from build123d import *
from OCP.BRepAlgoAPI import BRepAlgoAPI_Cut
from OCP.TopTools import TopTools_ListOfShape
from build123d.topology import SkipClean

# Parameters (mm, degrees)
BOSS_EXTRUDE1_DEPTH = 7.5
CUT_EXTRUDE1_DEPTH  = 3.2
CUT_EXTRUDE4_REACH  = 70.655
SKETCH5_W           = 3
SKETCH5_H           = 17
CUT_EXTRUDE5_REACH  = 70.655
SKETCH8_W           = 12
SKETCH8_H           = 37
CUT_EXTRUDE6_DEPTH  = 3.2
SKETCH10_W          = 10
SKETCH10_H          = 7.5
BOSS_EXTRUDE2_DEPTH = 27.486353186
SKETCH11_W          = 3
SKETCH11_H          = 7.5
CUT_EXTRUDE7_DEPTH  = 3.5
SKETCH12_W          = 2
SKETCH12_H          = 7.5
CUT_EXTRUDE8_DEPTH  = 4
SKETCH13_W          = 2
SKETCH13_H          = 7.5
CUT_EXTRUDE9_DEPTH  = 4
SKETCH14_W          = 7.5
SKETCH14_H          = 9.5
CUT_EXTRUDE10_DEPTH = 6
SKETCH15_W          = 1.5
SKETCH15_H          = 21
SKETCH15_H_2        = 1
CUT_EXTRUDE11_DEPTH = 1.5
SKETCH16_W          = 1.5
SKETCH16_H          = 7.5
CUT_EXTRUDE12_DEPTH = 35.486360958
CUT_EXTRUDE13_DEPTH = 6
SKETCH19_W          = 17.5
SKETCH19_H          = 32
BOSS_EXTRUDE3_DEPTH = 7.5
CUT_EXTRUDE14_DEPTH = 6
SKETCH20_W          = 18
SKETCH20_H          = 6
CUT_EXTRUDE15_DEPTH = 6
SKETCH21_W          = 20
SKETCH21_H          = 33
CUT_EXTRUDE16_DEPTH = 11
CUT_EXTRUDE17_DEPTH = 5
CUT_EXTRUDE18_DEPTH = 10
SKETCH23_W          = 50
SKETCH23_H          = 4
BOSS_EXTRUDE4_DEPTH = 15
SKETCH25_R          = 3.5
CUT_EXTRUDE19_DEPTH = 10


with BuildPart() as part:
    # Sketch1 → Boss-Extrude1 (new body)
    with BuildSketch(Plane.XY):
        with BuildLine():
            Line((-33, -47.5), (49, -47.5))
            Line((49, -47.5), (49, -29.5))
            Line((49, -29.5), (31.5, -29.5))
            Line((31.5, -29.5), (31.5, 2.5))
            Line((31.5, 2.5), (49, 2.5))
            Line((49, 2.5), (49, 47.5))
            Line((49, 47.5), (30, 47.5))
            Line((30, 47.5), (30, 30.5))
            Line((30, 30.5), (27, 30.5))
            Line((27, 30.5), (27, 47.5))
            Line((27, 47.5), (-49, 47.5))
            Line((-49, 47.5), (-49, -31.5))
            ThreePointArc((-49, -31.5), (-44.313708499, -42.813708499), (-33, -47.5))
        make_face()
    extrude(amount=BOSS_EXTRUDE1_DEPTH)

    # Sketch2 → Cut-Extrude1 (cut)
    with BuildSketch(Plane.XY.offset(7.5)):
        Polygon((30, 40), (31, 40), (31, 32.5), (36, 32.5), (36, 28.5), (38, 28.5), (38, 32.5), (48, 32.5), (48, 46.5), (38, 46.5), (38, 47.5), (36, 47.5), (36, 46.5), (31, 46.5), (31, 45), (30, 45), align=None)
        Polygon((-16, 40), (-15, 40), (-15, 32.5), (-10, 32.5), (-10, 28.5), (-8, 28.5), (-8, 32.5), (2, 32.5), (2, 46.5), (-8, 46.5), (-8, 47.5), (-10, 47.5), (-10, 46.5), (-15, 46.5), (-15, 45), (-16, 45), align=None)
        Polygon((7, 40), (8, 40), (8, 32.5), (13, 32.5), (13, 28.5), (15, 28.5), (15, 32.5), (25, 32.5), (25, 46.5), (15, 46.5), (15, 47.5), (13, 47.5), (13, 46.5), (8, 46.5), (8, 45), (7, 45), align=None)
    extrude(amount=-CUT_EXTRUDE1_DEPTH, mode=Mode.SUBTRACT)

    # Sketch5 → Cut-Extrude4 (cut, up to next)
    with BuildSketch(Plane.XY.offset(7.5), mode=Mode.PRIVATE) as cut_extrude4_sk1:
        with Locations((5.5, 39)):
            Rectangle(SKETCH5_W, SKETCH5_H)
    cut_extrude4_tool1 = extrude(cut_extrude4_sk1.sketch, amount=-CUT_EXTRUDE4_REACH, mode=Mode.PRIVATE) & part.part
    # Sketch5 → Cut-Extrude4 (cut, up to next)
    with BuildSketch(Plane.XY.offset(7.5), mode=Mode.PRIVATE) as cut_extrude4_sk2:
        with Locations((-17.5, 39)):
            Rectangle(SKETCH5_W, SKETCH5_H)
    cut_extrude4_tool2 = extrude(cut_extrude4_sk2.sketch, amount=-CUT_EXTRUDE4_REACH, mode=Mode.PRIVATE) & part.part
    add(cut_extrude4_tool1.solids().sort_by_distance((5.5, 39, 7.5))[0], mode=Mode.SUBTRACT)
    add(cut_extrude4_tool2.solids().sort_by_distance((-17.5, 39, 7.5))[0], mode=Mode.SUBTRACT)

    # Sketch8 → Cut-Extrude5 (cut, up to next)
    with BuildSketch(Plane.XY.offset(7.5), mode=Mode.PRIVATE) as cut_extrude5_sk1:
        with Locations((-43, 29)):
            Rectangle(SKETCH8_W, SKETCH8_H)
    cut_extrude5_tool1 = extrude(cut_extrude5_sk1.sketch, amount=-CUT_EXTRUDE5_REACH, mode=Mode.PRIVATE) & part.part
    add(cut_extrude5_tool1.solids().sort_by_distance((-43, 29, 7.5))[0], mode=Mode.SUBTRACT)

    # Sketch9 → Cut-Extrude6 (cut)
    with BuildSketch(Plane.XY.offset(7.5)):
        Polygon((-37, 20), (-36, 20), (-36, 12.5), (-31, 12.5), (-31, 8.5), (-29, 8.5), (-29, 12.5), (-19, 12.5), (-19, 26.5), (-29, 26.5), (-29, 30.5), (-31, 30.5), (-31, 26.5), (-36, 26.5), (-36, 25), (-37, 25), align=None)
    extrude(amount=-CUT_EXTRUDE6_DEPTH, mode=Mode.SUBTRACT)

    # Sketch10 → Boss-Extrude2 (add)
    with BuildSketch(Plane(origin=(0, 10.5, 0), x_dir=(1, 0, 0), z_dir=(0, 1, 0))):
        with Locations((-44, -3.75)):
            Rectangle(SKETCH10_W, SKETCH10_H)
    extrude(amount=BOSS_EXTRUDE2_DEPTH)

    # Sketch11 → Cut-Extrude7 (cut)
    with BuildSketch(Plane(origin=(0, 30.5, 0), x_dir=(1, 0, 0), z_dir=(0, 1, 0))):
        with Locations((-17.5, -3.75)):
            Rectangle(SKETCH11_W, SKETCH11_H)
        with Locations((5.5, -3.75)):
            Rectangle(SKETCH11_W, SKETCH11_H)
        with Locations((28.5, -3.75)):
            Rectangle(SKETCH11_W, SKETCH11_H)
    extrude(amount=-CUT_EXTRUDE7_DEPTH, mode=Mode.SUBTRACT)

    # Sketch12 → Cut-Extrude8 (cut)
    with BuildSketch(Plane(origin=(0, 10.5, 0), x_dir=(1, 0, 0), z_dir=(0, 1, 0))):
        with Locations((-38, -3.75)):
            Rectangle(SKETCH12_W, SKETCH12_H)
    extrude(amount=-CUT_EXTRUDE8_DEPTH, mode=Mode.SUBTRACT)

    # Sketch13 → Cut-Extrude9 (cut)
    with BuildSketch(Plane(origin=(0, 6.5, 0), x_dir=(1, 0, 0), z_dir=(0, 1, 0))):
        with Locations((-38, -3.75)):
            Rectangle(SKETCH13_W, SKETCH13_H)
    extrude(amount=-CUT_EXTRUDE9_DEPTH, mode=Mode.SUBTRACT)

    # Sketch14 → Cut-Extrude10 (cut)
    with BuildSketch(Plane.ZY.offset(37)):
        with Locations((3.75, 42.75)):
            Rectangle(SKETCH14_W, SKETCH14_H)
    extrude(amount=-CUT_EXTRUDE10_DEPTH, mode=Mode.SUBTRACT)

    # Sketch15 → Cut-Extrude11 (cut)
    with BuildSketch(Plane.XY.offset(7.5)):
        with Locations((-19.75, 37)):
            Rectangle(SKETCH15_W, SKETCH15_H)
        with Locations((1.25, 47)):
            Rectangle(SKETCH15_W, SKETCH15_H_2)
        with Locations((24.25, 47)):
            Rectangle(SKETCH15_W, SKETCH15_H_2)
        with Locations((47.25, 47)):
            Rectangle(SKETCH15_W, SKETCH15_H_2)
    extrude(amount=-CUT_EXTRUDE11_DEPTH, mode=Mode.SUBTRACT)


with BuildPart() as cut_extrude12_tool:
    # Sketch16 → Cut-Extrude12 (new body)
    with BuildSketch(Plane(origin=(0, 37.986353186, 0), x_dir=(1, 0, 0), z_dir=(0, 1, 0))):
        with Locations((-39.75, -3.75)):
            Rectangle(SKETCH16_W, SKETCH16_H)
    extrude(amount=-CUT_EXTRUDE12_DEPTH)


with BuildPart() as part_1:
    add(part.part)

    # Cut-Extrude12: cut by cut_extrude12_tool, with a tolerance
    cut_extrude12_stock = TopTools_ListOfShape()
    cut_extrude12_stock.Append(part_1.part.wrapped)
    cut_extrude12_tools = TopTools_ListOfShape()
    cut_extrude12_tools.Append(cut_extrude12_tool.part.wrapped)
    cut_extrude12_cut = BRepAlgoAPI_Cut()
    cut_extrude12_cut.SetArguments(cut_extrude12_stock)
    cut_extrude12_cut.SetTools(cut_extrude12_tools)
    cut_extrude12_cut.SetFuzzyValue(0.00001)
    cut_extrude12_cut.Build()
    add(Compound.cast(cut_extrude12_cut.Shape()).solids(), mode=Mode.REPLACE)

    # Sketch18 → Cut-Extrude13 (cut)
    with SkipClean():  # the faces are left unmerged after this step: merging them gives an invalid solid
        with BuildSketch(Plane.XY.offset(7.5)):
            Polygon((23.5, 5.5), (23.5, 1.5), (47, 1.5), (47, 24.5), (49, 24.5), (49, 26.5), (47, 26.5), (23.5, 26.5), (23.5, 8.5), (17, 8.5), (17, 5.5), align=None)
        extrude(amount=-CUT_EXTRUDE13_DEPTH, mode=Mode.SUBTRACT)

    # Sketch19 → Boss-Extrude3 (add)
    with SkipClean():  # the faces are left unmerged after this step: merging them gives an invalid solid
        with BuildSketch(Plane(origin=(0, 0, 0), x_dir=(-1, 0, 0), z_dir=(0, 0, -1))):
            with Locations((-40.25, -13.5)):
                Rectangle(SKETCH19_W, SKETCH19_H)
        extrude(amount=-BOSS_EXTRUDE3_DEPTH)

    # Sketch18_2 → Cut-Extrude14 (cut)
    with SkipClean():  # the faces are left unmerged after this step: merging them gives an invalid solid
        with BuildSketch(Plane.XY.offset(7.5)):
            Polygon((23.5, 5.5), (23.5, 1.5), (47, 1.5), (47, 24.5), (49, 24.5), (49, 26.5), (47, 26.5), (23.5, 26.5), (23.5, 8.5), (17, 8.5), (17, 5.5), align=None)
        extrude(amount=-CUT_EXTRUDE14_DEPTH, mode=Mode.SUBTRACT)

    # Sketch20 → Cut-Extrude15 (cut)
    with SkipClean():  # the faces are left unmerged after this step: merging them gives an invalid solid
        with BuildSketch(Plane.XY.offset(7.5)):
            with Locations((38, -1.5)):
                Rectangle(SKETCH20_W, SKETCH20_H)
        extrude(amount=-CUT_EXTRUDE15_DEPTH, mode=Mode.SUBTRACT)

    # Sketch21 → Cut-Extrude16 (cut)
    with SkipClean():  # the faces are left unmerged after this step: merging them gives an invalid solid
        with BuildSketch(Plane.XY.offset(7.5)):
            with Locations((39, -21)):
                Rectangle(SKETCH21_W, SKETCH21_H)
        extrude(amount=-CUT_EXTRUDE16_DEPTH, mode=Mode.SUBTRACT)

    # Sketch3 → Cut-Extrude17 (cut)
    with SkipClean():  # the faces are left unmerged after this step: merging them gives an invalid solid
        with BuildSketch(Plane.XZ.offset(47.5)):
            with BuildLine():
                Line((34.25, 7.5), (46.25, 7.5))
                ThreePointArc((46.25, 7.5), (40.25, 1.5), (34.25, 7.5))
            make_face()
        extrude(amount=-CUT_EXTRUDE17_DEPTH, mode=Mode.SUBTRACT)

    # Sketch22 → Cut-Extrude18 (cut)
    with SkipClean():  # the faces are left unmerged after this step: merging them gives an invalid solid
        with BuildSketch(Plane.XZ.offset(42.5)):
            with BuildLine():
                Line((37.25, 7.5), (43.25, 7.5))
                ThreePointArc((43.25, 7.5), (40.25, 4.5), (37.25, 7.5))
            make_face()
        extrude(amount=-CUT_EXTRUDE18_DEPTH, mode=Mode.SUBTRACT)

    # Sketch23 → Boss-Extrude4 (add)
    with SkipClean():  # the faces are left unmerged after this step: merging them gives an invalid solid
        with BuildSketch(Plane(origin=(0, 0, 0), x_dir=(-1, 0, 0), z_dir=(0, 0, -1))):
            with Locations((6, -45.5)):
                Rectangle(SKETCH23_W, SKETCH23_H)
        extrude(amount=BOSS_EXTRUDE4_DEPTH)

    # Sketch25 → Cut-Extrude19 (cut)
    with SkipClean():  # the faces are left unmerged after this step: merging them gives an invalid solid
        with BuildSketch(Plane(origin=(0, -47.5, 0), x_dir=(-1, 0, 0), z_dir=(0, -1, 0))):
            with Locations(Location((-1, 7.5, 0), (0, 0, 180))):
                Circle(SKETCH25_R)
        extrude(amount=-CUT_EXTRUDE19_DEPTH, mode=Mode.SUBTRACT)


solid = part_1.part
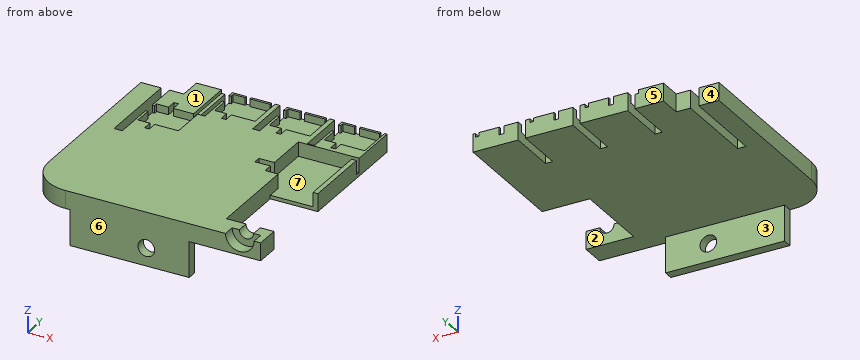
Design review of the part built by this model. Coordinates are the model's own, in mm. Face numbers are marked on the shaded views. A direction names the side the tool comes from. Give positions to 0.01 mm unless a question says otherwise; leave off trailing zeros. Loops run counter-clockwise (first coordinate to the right, second up) from the corner with the lowest first, then second, coordinate; pieces in that order, holes last. Notation, with made-up numbers: (24, 8) - (67, 8) arc R25 ccw to (67, 27) - close; hole circle Ø1 at (-40, 69.25). An arc over 180 degrees is marked (long way). Write item = value, one per line.
1) Take a section at D-D on y = -24. State the section outline as (x, z) points, and give its area (3 significant figures).
Result sheet:
outline = (-49, 0) - (29, 0) - (29, 7.5) - (-49, 7.5) - close
area = 585 mm2
2) Take a section at B-B on z = -7.5. State the section outline as (x, y) points, and give its area (3 significant figures).
Result sheet:
outline = (-31, -47.5) - (-2.5, -47.5) - (-2.5, -43.5) - (-31, -43.5) - close; (4.5, -47.5) - (19, -47.5) - (19, -43.5) - (4.5, -43.5) - close
area = 172 mm2
3) Take a section at C-C on y = 18. State the section outline as (x, z) points.
Result sheet:
outline = (-49, 0) - (-40.5, 0) - (-40.5, 7.5) - (-49, 7.5) - close; (-37, 0) - (49, 0) - (49, 7.5) - (47, 7.5) - (47, 1.5) - (23.5, 1.5) - (23.5, 7.5) - (-19, 7.5) - (-19, 4.3) - (-36, 4.3) - (-36, 7.5) - (-37, 7.5) - close
4) Tool access review of the marked faces 1, 2, 3, 4 and 5: name each direction out of +Z, -Z, +X, -X, +Y, -Y from which nothing blocks a thin tool from reaching the whole face with its end or side.
Result sheet:
face_1 = +Z, +X, -X, +Y, -Y
face_2 = +Z, -Z, +X
face_3 = -Z, +X, -X, +Y
face_4 = +Z, -Z, -X, +Y
face_5 = +Z, -Z, +X, -X, +Y
5) To check wall thickness, follow line 1 (X direction, y = 3, z = 4.25); line 2 (Z direction, x = 1, y = -44.45); line 3 (Y direction, x = -3, z = -6.25). State the ranges of each line that lie inside material, in increasing order.
Result sheet:
line_1 = -49 to -40.5, -37 to 23.5, 47 to 49
line_2 = -15 to -11, -4 to 7.5
line_3 = -47.5 to -43.5
6) Clearance check with flat-ended pins moving along their axes: pin 1 Ø3.5 at (x, z) = (28.5, 3) entering from +Y; pin 2 Ø5.5 at (x, y) = (40.5, 42.5) entering from +Z; pin 3 Ø1.8 at (x, z) = (-34.5, 4) entering from +Y; pin 4 Ø10 at (x, y) = (7, 23.5) entering from -Z. State where each tip first meets the part, or that it passes through.
Result sheet:
pin_1 = 47.5
pin_2 = 4.3
pin_3 = 38
pin_4 = 0
7) Take a section at A-A on x = 40.25. State the section outline as (y, z) points.
Result sheet:
outline = (-47.5, 0) - (-37.5, 0) - (-37.5, 4.5) - (-42.5, 4.5) - (-42.5, 1.5) - (-47.5, 1.5) - close; (-4.5, 0) - (47.5, 0) - (47.5, 7.5) - (46.5, 7.5) - (46.5, 4.3) - (32.5, 4.3) - (32.5, 7.5) - (26.5, 7.5) - (26.5, 1.5) - (-4.5, 1.5) - close
8) Draft analysis for pull direction X (two halves, no side actions). For the marked faces 6 and 7, state which applies: +X half, -X half, draft (parallel to the pull), parting line (faces both ways), or undercut.
Result sheet:
face_6 = draft
face_7 = undercut
